from build123d import *

# Parameters (mm, degrees)
BOSS_EXTRUDE1_DEPTH     = 12.7
SKETCH4_R               = 3.5
CUT_EXTRUDE1_DEPTH      = 530.352708504
CUT_EXTRUDE2_DEPTH      = 530.352708504
CUT_EXTRUDE2_DEPTH_BACK = 530.352708504
SKETCH5_R               = 3.5


with BuildPart() as part:
    # Sketch2 → Boss-Extrude1 (new body)
    with BuildSketch(Plane.XY):
        with BuildLine():
            Line((-492, -87), (492, -87))
            ThreePointArc((492, -87), (513.213203436, -78.213203436), (522, -57))
            Line((522, -57), (522, 57))
            ThreePointArc((522, 57), (513.213203436, 78.213203436), (492, 87))
            Line((492, 87), (-492, 87))
            ThreePointArc((-492, 87), (-513.213203436, 78.213203436), (-522, 57))
            Line((-522, 57), (-522, -57))
            ThreePointArc((-522, -57), (-513.213203436, -78.213203436), (-492, -87))
        make_face()
        with BuildLine():
            Line((-492, -69), (492, -69))
            ThreePointArc((492, -69), (500.485281374, -65.485281374), (504, -57))
            Line((504, -57), (504, 57))
            ThreePointArc((504, 57), (500.485281374, 65.485281374), (492, 69))
            Line((492, 69), (-492, 69))
            ThreePointArc((-492, 69), (-500.485281374, 65.485281374), (-504, 57))
            Line((-504, 57), (-504, -57))
            ThreePointArc((-504, -57), (-500.485281374, -65.485281374), (-492, -69))
        make_face(mode=Mode.SUBTRACT)
    extrude(amount=BOSS_EXTRUDE1_DEPTH)

    # Sketch4 → Cut-Extrude1 (cut, through all)
    with BuildSketch(Plane.XY.offset(12.7)):
        with Locations((-507.727922061, 72.727922061)):
            Circle(SKETCH4_R)
        with Locations((-507.727922061, -72.727922061)):
            Circle(SKETCH4_R)
        with Locations((-250.5, -78)):
            Circle(SKETCH4_R)
        with Locations((-250.5, 78)):
            Circle(SKETCH4_R)
        with Locations((250.5, 78)):
            Circle(SKETCH4_R)
        with Locations((250.5, -78)):
            Circle(SKETCH4_R)
        with Locations((507.727922061, 72.727922061)):
            Circle(SKETCH4_R)
        with Locations((507.727922061, -72.727922061)):
            Circle(SKETCH4_R)
    extrude(amount=-CUT_EXTRUDE1_DEPTH, mode=Mode.SUBTRACT)

    # Sketch5 → Cut-Extrude2 (cut, two sides: drawn at the far end of the back side and taken through both)
    with BuildSketch(Plane.XY.offset(12.7).offset(-CUT_EXTRUDE2_DEPTH_BACK)):
        with Locations((-379.113961031, 78)):
            Circle(SKETCH5_R)
        with Locations((-513, 0)):
            Circle(SKETCH5_R)
        with Locations((-379.113961031, -78)):
            Circle(SKETCH5_R)
        with Locations((0, -78)):
            Circle(SKETCH5_R)
        with Locations((0, 78)):
            Circle(SKETCH5_R)
        with Locations((379.113961031, 78)):
            Circle(SKETCH5_R)
        with Locations((379.113961031, -78)):
            Circle(SKETCH5_R)
        with Locations((513, 0)):
            Circle(SKETCH5_R)
    extrude(amount=CUT_EXTRUDE2_DEPTH + CUT_EXTRUDE2_DEPTH_BACK, mode=Mode.SUBTRACT)


solid = part.part
Geometry check sheet. Reference: the model listing, model coordinates, mm. Round coordinates to 2 decimals unless told otherwise and drop trailing zeros. Loops run counter-clockwise (first coordinate to the right, second up) from the corner with the lowest first, then second, coordinate; pieces in that order, holes last. Notation, with made-up numbers: (-6, 84.5) - (12, 84.5) arc R18 ccw to (12, 95.5) - close; hole circle Ø11 at (70.25, 52). An arc over 180 degrees is marked (long way). One line per question, with ' | ' between items. Start each with the question number.
1. Cross-section at A-A on x = -139.5. Record the cut outline in (y, z), then the cut area to 3 significant figures.
2. Cross-section at B-B on y = 15. Record the cut outline in (x, z), then the cut area to 3 significant figures.
3. Scan lines: line 1 (Y direction, x = 250.5, z = 3); line 2 (Y direction, x = 223, z = 10.75); line 3 (X direction, y = 35.5, z = 11.5). Record each from-to range of solid material in increasing order. Write a range as [from, to].
4. Depth check by flat-ended pin: pin 1 (5.5 mm diameter, centred on x = 250.5, y = 78, fed in from +Z); pin 2 (1.5 mm diameter, centred on y = -63.5, z = 6, fed in from +X); pin 3 (2 mm diameter, centred on y = -65.5, z = 7, fed in from +X). Enter the tip coordinate at first touch or a pass-through.
5. Cross-section at C-C on z = 2.25. State how many separate pieces and enclosed holes the cut face has, then the cut area to 3 significant figures.
Taken from the geometry:
1) outline: (-87, 0) - (-69, 0) - (-69, 12.7) - (-87, 12.7) - close; (69, 0) - (87, 0) - (87, 12.7) - (69, 12.7) - close | area: 457 mm²
2) outline: (-522, 0) - (-504, 0) - (-504, 12.7) - (-522, 12.7) - close; (504, 0) - (522, 0) - (522, 12.7) - (504, 12.7) - close | area: 457 mm²
3) line 1: [-87, -81.5], [-74.5, -69], [69, 74.5], [81.5, 87] | line 2: [-87, -69], [69, 87] | line 3: [-522, -504], [504, 522]
4) pin 1: through | pin 2: x = 521.44 | pin 3: x = 521.05
5) separate pieces: 1 | enclosed holes: 17 | area: 41,300 mm²
